The listing builds one solid part. Answer for the finished solid, in the listing's coordinates (mm). A direction names the side the tool comes from. Coordinates: 2 decimals unless noted, no trailing zeros. Order: outer loops, then holes, each group sorted by start corner. A loop starts at its lowest first (then second) coordinate and runs counter-clockwise, first axis right, second up. Notation, with made-up numbers: (86.5, 74.25) -> (130.5, 74.25) arc R23 cw to (130.5, 97.25) -> close; hole circle Ø8 at (-16, 12). An arc over 180 degrees is marked (long way). Return JSON: item names as keys, results as strings.
from build123d import *

# Parameters (mm, degrees)
SKETCH1_R           = 12.5
BOSS_EXTRUDE1_DEPTH = 51.8
SKETCH2_R           = 3.5
BOSS_EXTRUDE2_DEPTH = 2.38
SKETCH3_R           = 1.5
CUT_EXTRUDE1_DEPTH  = 5
SKETCH4_R           = 2
CUT_EXTRUDE2_DEPTH  = 57.990985252


with BuildPart() as part:
    # Sketch1 → Boss-Extrude1 (new body)
    with BuildSketch(Plane.XY):
        with Locations(Location((0, 0, 0), (0, 0, 180))):
            Circle(SKETCH1_R)
    extrude(amount=BOSS_EXTRUDE1_DEPTH)

    # Sketch2 → Boss-Extrude2 (add)
    with BuildSketch(Plane(origin=(0, 0, 0), x_dir=(-1, 0, 0), z_dir=(0, 0, -1))):
        Circle(SKETCH2_R)
    extrude(amount=BOSS_EXTRUDE2_DEPTH)

    # Sketch3 → Cut-Extrude1 (cut)
    with BuildSketch(Plane(origin=(0, 0, 0), x_dir=(-1, 0, 0), z_dir=(0, 0, -1))):
        with Locations((8.5, 0)):
            Circle(SKETCH3_R)
        with Locations((-8.5, 0)):
            Circle(SKETCH3_R)
    extrude(amount=-CUT_EXTRUDE1_DEPTH, mode=Mode.SUBTRACT)

    # Sketch4 → Cut-Extrude2 (cut, through all)
    with BuildSketch(Plane(origin=(0, 0, -2.38), x_dir=(-1, 0, 0), z_dir=(0, 0, -1))):
        Circle(SKETCH4_R)
    extrude(amount=-CUT_EXTRUDE2_DEPTH, mode=Mode.SUBTRACT)


solid = part.part
1. The part is cut by section B-B on y = 0. Give the vertices of the cut face in (x, z), and give its area (3 significant figures).
Answer block:
{"outline": "(-12.5, 0) -> (-10, 0) -> (-10, 5) -> (-7, 5) -> (-7, 0) -> (-3.5, 0) -> (-3.5, -2.38) -> (-2, -2.38) -> (-2, 51.8) -> (-12.5, 51.8) -> close; (2, -2.38) -> (3.5, -2.38) -> (3.5, 0) -> (7, 0) -> (7, 5) -> (10, 5) -> (10, 0) -> (12.5, 0) -> (12.5, 51.8) -> (2, 51.8) -> close", "area": "1,060 mm2"}
2. The part is cut by section C-C on z = 13.5. Give the vertices of the cut face in (x, y), and give its area (3 significant figures).
Answer block:
{"outline": "circle Ø25 at (0, 0); hole circle Ø4 at (0, 0)", "area": "478 mm2"}
3. Determine the mould class of faces 3 (the face through (-3, 3, 0)), 4 (the face through (-8, 0, 5)), 5 (the face through (0, -2, 24)), 6 (the face through (-3.233, -1.341, -1.173)) for opening direction Y: pulls with the +Y half, pulls with the -Y half, needs draft (parallel to the pull), parting line crosses it, or undercut.
Answer block:
{"face 3": "needs draft", "face 4": "undercut", "face 5": "undercut", "face 6": "parting line crosses it"}
4. The part is cut by section D-D on x = -8.5. Give the vertices of the cut face in (y, z), and give its area (3 significant figures).
Answer block:
{"outline": "(-9.17, 0) -> (-1.5, 0) -> (-1.5, 5) -> (1.5, 5) -> (1.5, 0) -> (9.17, 0) -> (9.17, 51.8) -> (-9.17, 51.8) -> close", "area": "935 mm2"}
5. Consider line 1 (Y direction, x = 0, z = 13); line 2 (Z direction, x = -6.75, y = 0.75); line 3 (Y direction, x = -0.75, z = 18). Determine where each line is inside the solid, lowest interval first. Write a range as from..to.
Answer block:
{"line 1": "y = -12.5..-2, 2..12.5", "line 2": "z = 0..51.8", "line 3": "y = -12.48..-1.85, 1.85..12.48"}
6. Each of these flat-tipped pins is pushed along its axis until it touches: pin 1 Ø6 at (x, z) = (7, 7.5) entering from -Y; pin 2 Ø1 at (x, y) = (1.5, 0.5) entering from -Z; pin 3 Ø3.5 at (x, y) = (8, 0.5) entering from -Z; pin 4 Ø1 at (y, z) = (8, 20.5) entering from +X. Where does it stop, or does it pass through?
Answer block:
{"pin 1": "stops at y = -11.84", "pin 2": "stops at z = -2.38", "pin 3": "stops at z = 0", "pin 4": "stops at x = 10"}
7. The part is cut by section A-A on x = 0. Give the vertices of the cut face in (y, z), and give its area (3 significant figures).
Answer block:
{"outline": "(-12.5, 0) -> (-3.5, 0) -> (-3.5, -2.38) -> (-2, -2.38) -> (-2, 51.8) -> (-12.5, 51.8) -> close; (2, -2.38) -> (3.5, -2.38) -> (3.5, 0) -> (12.5, 0) -> (12.5, 51.8) -> (2, 51.8) -> close", "area": "1,090 mm2"}
8. For faces 1 (the face through (-2, -2, -2.38)), 2 (the face through (10, 0, 2)), determine the directions among +Z, -Z, +X, -X, +Y, -Y from which every point of the face is accessible in a straight line to the end or side of a thin tool.
Answer block:
{"face 1": "-Z, +X, -X, +Y, -Y", "face 2": "-Z"}
